```python
from build123d import *

# Parameters (mm, degrees)
PAD_DEPTH = 25


with BuildPart() as part:
    # Sketch → Pad (new body)
    with BuildSketch(Plane.XY):
        with BuildLine():
            Line((-6, 18.103857), (-6, 2))
            ThreePointArc((-6, 2), (-5.414214, 0.585786), (-4, 0))
            Line((-4, 0), (4, 0))
            ThreePointArc((4, 0), (5.414214, 0.585786), (6, 2))
            Line((6, 2), (6, 18.103857))
            ThreePointArc((6, 18.103857), (3.571924, 20.479424), (1.25, 18))
            Line((1.6, 10), (1.25, 18))
            Line((-1.6, 10), (1.6, 10))
            Line((-1.25, 18), (-1.6, 10))
            ThreePointArc((-1.25, 18), (-3.571924, 20.479424), (-6, 18.103857))
        make_face()
    extrude(amount=PAD_DEPTH)


solid = part.part
```
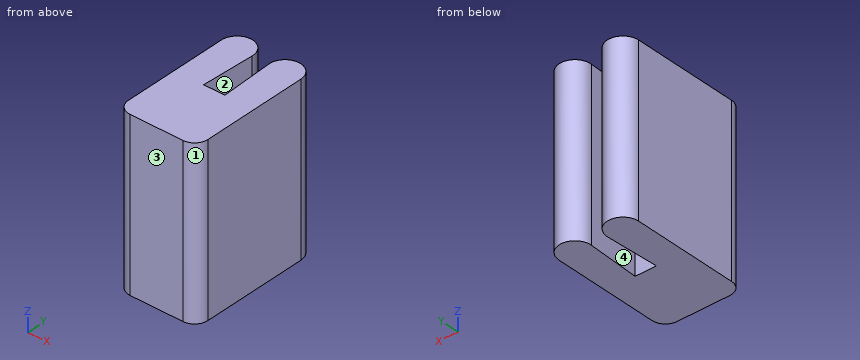
The listing builds one solid part. Answer for the finished solid, in the listing's coordinates (mm). Face numbers are marked on the shaded views. Coordinates: 2 decimals unless noted, no trailing zeros. Write each loop counter-clockwise with the first axis right and the second up, starting at its lowest first coordinate (ties: lowest second). Pieces come first, ordered by that corner, then holes. Notation, with made-up numbers: (39.5, 74.5) - (86.5, 74.5) arc R13 cw to (86.5, 83.5) - close; hole circle Ø7 at (61, 31). An arc over 180 degrees is marked (long way). Return JSON: item names as keys, results as strings. Group by question number.
Q1. The part is cut by section B-B on z = 2.25. Write down the section's boundary in (x, y), and give its area (3 significant figures).
Q2. The part is cut by section D-D on x = -2.25. Write down the section's boundary in (y, z), and give its area (3 significant figures).
Q3. For a pull along X with two mould halves and no side action, classify the marked faces 1, 2, 3 and 4 as +X half, -X half, draft (parallel to the pull), parting line (faces both ways), or undercut.
Q4. The part is cut by section C-C on y = 15.5. Write down the section's boundary in (x, z).
Q5. The part is cut by section A-A on y = 10.75. Write down the section's boundary in (x, z), and give its area (3 significant figures).
Q6. Find the intervals of material crossed by line 1 along Y through (x, z) = (-0.5, 11.5); line 2 along X through (y, z) = (11.5, 19.5); line 3 along X through (y, z) = (14.75, 6.5), in increasing order. Write a range as [from, to].
Q7. Flat-ended cylindrical pins translate along their axes: pin 1 Ø2.5 at (x, z) = (0.5, 9) entering from +Y; pin 2 Ø1.5 at (x, z) = (1.5, 15) entering from +Y. Find the tip coordinate at first contact, or state that the pin passes through.
Evaluation:
{
 "1": {"outline": "(-6, 2) arc R2 ccw to (-4, 0) - (4, 0) arc R2 ccw to (6, 2) - (6, 18.1) arc R2.38 ccw (long way) to (1.25, 18) - (1.6, 10) - (-1.6, 10) - (-1.25, 18) arc R2.38 ccw (long way) to (-6, 18.1) - close", "area": "210 mm2"},
 "2": {"outline": "(0, 0) - (20.04, 0) - (20.04, 25) - (0, 25) - close", "area": "501 mm2"},
 "3": {"face 1": "+X half", "face 2": "undercut", "face 3": "draft", "face 4": "undercut"},
 "4": {"outline": "(-6, 0) - (-1.36, 0) - (-1.36, 25) - (-6, 25) - close; (1.36, 0) - (6, 0) - (6, 25) - (1.36, 25) - close"},
 "5": {"outline": "(-6, 0) - (-1.57, 0) - (-1.57, 25) - (-6, 25) - close; (1.57, 0) - (6, 0) - (6, 25) - (1.57, 25) - close", "area": "222 mm2"},
 "6": {"line 1": "y = [0, 10]", "line 2": "x = [-6, -1.53], [1.53, 6]", "line 3": "x = [-6, -1.39], [1.39, 6]"},
 "7": {"pin 1": "stops at y = 19.56", "pin 2": "stops at y = 20.04"}
}
